Drawing for the job (mm, zero at the part's lowest x, y, z). Give positions to 0.01 mm unless a question says otherwise; leave off trailing zeros. Loops run counter-clockwise (first coordinate to the right, second up) from the corner with the lowest first, then second, coordinate; pieces in that order, holes last. Notation, with made-up numbers: (26, 42) -> (31, 42) arc R19 ccw to (31, 63) -> close; hole circle Ø10 at (24, -31). An arc over 180 degrees is marked (long way). Write item = value, one per line.
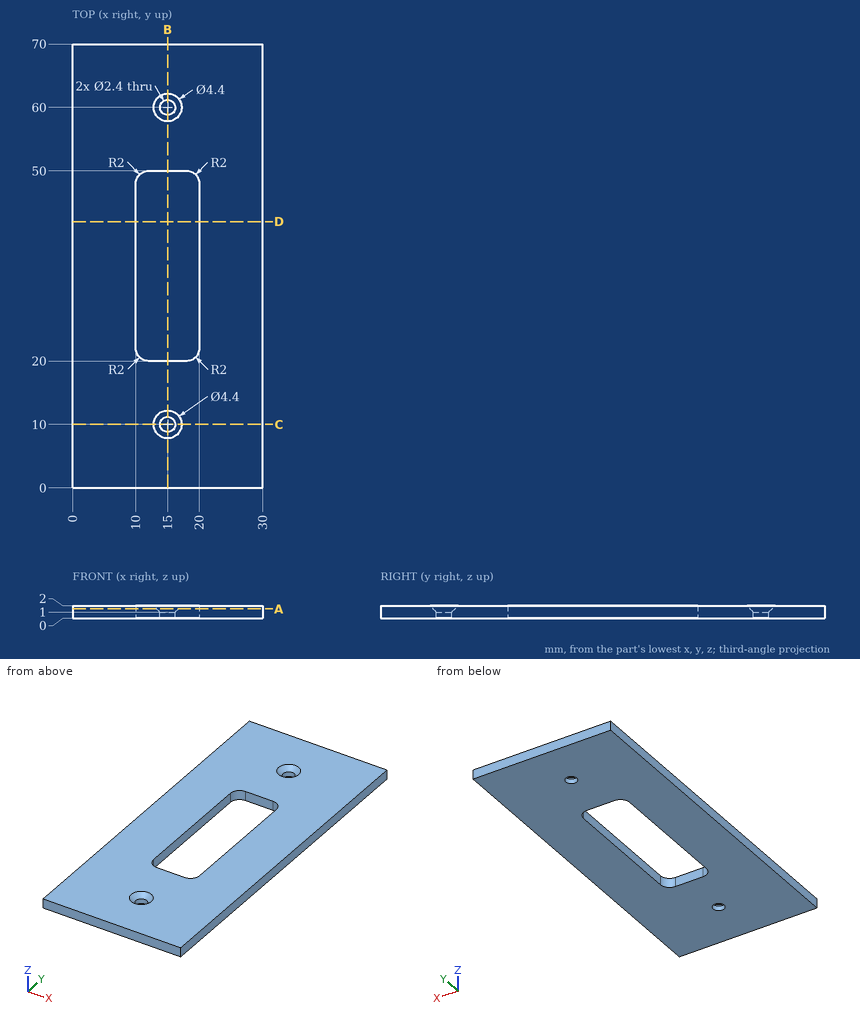
1) Drill centre lines: line 1 along Y through (x, z) = (15, 0.55); line 2 along X through (y, z) = (60, 0.75); line 3 along X through (y, z) = (41.5, 0.1). Where is each one in solid material? Low to high. Write a range as [from, to].
Resolved:
line_1 = [0, 8.8], [11.2, 20], [50, 58.8], [61.2, 70]
line_2 = [0, 13.8], [16.2, 30]
line_3 = [0, 10], [20, 30]
2) Drop a flat-ended pin along its axis: P1, Ø2, axis at x = 15, y = 10, coming from the -Z side. Give the stop position or say it passes through.
Resolved:
P1 = through
3) Slice it at A-A, the plane z = 1.5. List the corners of the cut face in (x, y).
Resolved:
outline = (0, 0) -> (30, 0) -> (30, 70) -> (0, 70) -> close; hole (10, 22) arc R2 ccw to (12, 20) -> (18, 20) arc R2 ccw to (20, 22) -> (20, 48) arc R2 ccw to (18, 50) -> (12, 50) arc R2 ccw to (10, 48) -> close; hole circle Ø3.4 at (15, 10); hole circle Ø3.4 at (15, 60)
4) Slice it at D-D, the plane y = 42. List the corners of the cut face in (x, z).
Resolved:
outline = (0, 0) -> (10, 0) -> (10, 2) -> (0, 2) -> close; (20, 0) -> (30, 0) -> (30, 2) -> (20, 2) -> close
5) Slice it at C-C, the plane y = 10. List the corners of the cut face in (x, z).
Resolved:
outline = (0, 0) -> (13.8, 0) -> (13.8, 1) -> (12.8, 2) -> (0, 2) -> close; (16.2, 0) -> (30, 0) -> (30, 2) -> (17.2, 2) -> (16.2, 1) -> close
6) Slice it at B-B, the plane x = 15. List the corners of the cut face in (y, z), and give its area (3 significant figures).
Resolved:
outline = (0, 0) -> (8.8, 0) -> (8.8, 1) -> (7.8, 2) -> (0, 2) -> close; (11.2, 0) -> (20, 0) -> (20, 2) -> (12.2, 2) -> (11.2, 1) -> close; (50, 0) -> (58.8, 0) -> (58.8, 1) -> (57.8, 2) -> (50, 2) -> close; (61.2, 0) -> (70, 0) -> (70, 2) -> (62.2, 2) -> (61.2, 1) -> close
area = 68.4 mm²
